```python
from build123d import *

# Parameters (mm, degrees)
F0_W     = 70
F0_H     = 40
F1_DEPTH = 8
F2_W     = 30
F2_H     = 40
F3_DEPTH = 25
F4_R     = 9.5
F5_DEPTH = 40
F7_D     = 5
F7_DEPTH = 15
F7_TIP   = 1.5021515476
F9_D     = 9
F9_DEPTH = 15
F9_TIP   = 2.7038727856


with BuildPart() as f1:
    # F0 (on Front) → F1 (new body)
    with BuildSketch(Plane.XZ):
        with Locations((35, 20)):
            Rectangle(F0_W, F0_H)
    extrude(amount=F1_DEPTH)

    # F2 (on face) → F3 (join)
    with BuildSketch(Plane.XZ.offset(8)):
        with Locations((15, 20)):
            Rectangle(F2_W, F2_H)
    extrude(amount=F3_DEPTH)

    # F4 (on face) → F5 (cut)
    with BuildSketch(Plane(origin=(0, 0, 0), x_dir=(1, 0, 0), z_dir=(0, 0, -1))):
        with Locations((15, 19)):
            Circle(F4_R)
    extrude(amount=-F5_DEPTH, mode=Mode.SUBTRACT)

    # F7
    with Locations(Plane(origin=(0, 0, 0), x_dir=(0, -1, 0), z_dir=(-1, 0, 0))):
        with Locations((19, 32), (19, 8)):
            Hole(F7_D / 2, depth=F7_DEPTH)
            with Locations((0, 0, -(F7_DEPTH + F7_TIP / 2))):  # 118° drill point
                Cone(0, F7_D / 2, F7_TIP, mode=Mode.SUBTRACT)

    # F9
    with Locations(Plane.XZ.offset(8)):
        with Locations((50, 20)):
            Hole(F9_D / 2, depth=F9_DEPTH)
            with Locations((0, 0, -(F9_DEPTH + F9_TIP / 2))):  # 118° drill point
                Cone(0, F9_D / 2, F9_TIP, mode=Mode.SUBTRACT)


solid = f1.part
```
Model file for the job. Use its own axes, mm. A direction names the side the tool comes from. Give positions to 0.01 mm unless a question says otherwise; leave off trailing zeros. Write each loop counter-clockwise with the first axis right and the second up, starting at its lowest first coordinate (ties: lowest second). Pieces come first, ordered by that corner, then holes. Notation, with made-up numbers: (0, 23.5) - (23, 23.5) arc R22 cw to (23, 57.5) - close; hole circle Ø2 at (36.25, -10.75). An arc over 180 degrees is marked (long way). One line per question, with ' | ' between items. Start each with the question number.
(1) Two-plate mould, pull along X, no slides. Class faces 4 (the face through (30, -20, 20)), 5 (the face through (0, -16, 20)), 6 (the face through (35, 0, 20)), 7 (the face through (23.776, -15.361, 19.72)): +X half, -X half, draft (parallel to the pull), parting line (faces both ways), or undercut.
(2) Slice it at A-A on z = 20. Write the cut outline in (x, y), plus the area to 3 significant figures.
(3) Wall check: line 1 along Z through (x, y) = (1.3, -19); line 2 along Y through (x, z) = (1, 8); line 3 along Y through (x, z) = (15, 14). Give the ranges that are in metal, low to high. Write a range as from..to.
(4) Pin check, flat tips, straight feed: P1, Ø12, axis at y = -17.5, z = 6, coming from the -X side; P2, Ø8, axis at y = -27, z = 15.5, coming from the +X side; P3, Ø20, axis at x = 55.5, z = 24.5, coming from the -Y side. Stop position of each tip, or through.
(5) Slice it at D-D on z = 26. Write the cut outline in (x, y), plus the area to 3 significant figures.
(6) Slice it at B-B on x = 15. Write the cut outline in (y, z).
(7) Slice it at C-C on y = -19. Write the cut outline in (x, z), plus the area to 3 significant figures.
(8) 3-axis set-ups, long thin cutter, end or side, ignore diameter. For faces 1 (the face through (27, -13, 40)), 2 (the face through (2.96, -16.69, 7.04)), 3 (the face through (45, -8, 20)): which of +Z, -Z, +X, -X, +Y, -Y reach the whole face in a straight line?
Results below:
1) face 4: +X half | face 5: -X half | face 6: draft | face 7: undercut
2) outline: (0, -33) - (30, -33) - (30, -8) - (45.5, -8) - (45.5, 0) - (0, 0) - close; (54.5, -8) - (70, -8) - (70, 0) - (54.5, 0) - close; hole circle Ø19 at (15, -19) | area: 954 mm^2
3) line 1: 0..5.5, 10.5..29.5, 34.5..40 | line 2: -33..-21.5, -16.5..0 | line 3: -33..-28.5, -9.5..0
4) P1: x = 0 | P2: x = 30 | P3: y = -8
5) outline: (0, -33) - (30, -33) - (30, -8) - (70, -8) - (70, 0) - (0, 0) - close; hole circle Ø19 at (15, -19) | area: 1,030 mm^2
6) outline: (-33, 0) - (-28.5, 0) - (-28.5, 40) - (-33, 40) - close; (-9.5, 0) - (0, 0) - (0, 40) - (-9.5, 40) - close
7) outline: (0, 0) - (5.5, 0) - (5.5, 5.5) - (0, 5.5) - close; (0, 10.5) - (5.5, 10.5) - (5.5, 29.5) - (0, 29.5) - close; (0, 34.5) - (5.5, 34.5) - (5.5, 40) - (0, 40) - close; (24.5, 0) - (30, 0) - (30, 40) - (24.5, 40) - close | area: 385 mm^2
8) face 1: +Z, +X, -X, +Y, -Y | face 2: -X | face 3: +Z, -Z, +X, -Y
